Check sheet for the modelled part. Datum: model origin and axes. Units: mm. Face numbers are marked on the shaded views. A direction names the side the tool comes from. Round coordinates to 2 decimals unless told otherwise and drop trailing zeros. Loops run counter-clockwise (first coordinate to the right, second up) from the corner with the lowest first, then second, coordinate; pieces in that order, holes last. Notation, with made-up numbers: (-28.5, -39.75) -> (-9.5, -39.75) arc R5 ccw to (-9.5, -30.75) -> close; hole circle Ø6 at (11, 80.5). An arc over 180 degrees is marked (long way). One line per item, written item: value. Start each with the question number.
1. Material ranges on L1, parallel to X at y = -12.5, z = 43.5; L2, parallel to Y at x = 9, z = -55.5, recorded low to high.
2. Go/stop test with flat-tipped pins: pin 1 (1 mm diameter, centred on x = -9, y = 0, fed in from -Z); pin 2 (7.5 mm diameter, centred on y = 3.5, z = 45.5, fed in from -X); pin 3 (20.5 mm diameter, centred on x = -6.5, z = 53, fed in from -Y). Record where each tip stops, or that it passes through.
3. Cross-section at D-D on y = 7.5. Record the cut outline in (x, z), then the cut area to 3 significant figures.
4. Cross-section at B-B on y = -4. Record the cut outline in (x, z).
5. Cross-section at A-A on x = 0. Record the cut outline in (y, z), then the cut area to 3 significant figures.
6. Set-up check for the marked faces 1, 2, 3, 4 and 5: record each of +Z, -Z, +X, -X, +Y, -Y from which the full face is reachable in a straight line by a thin tool's end or side.
7. Cross-section at C-C on y = 17.5. Record the cut outline in (x, z).
8. Release check for a two-part mould opening along Z. For the marked faces 6, 7 and 8 record: +Z half, -Z half, draft (parallel to the pull), parting line (faces both ways), or undercut.
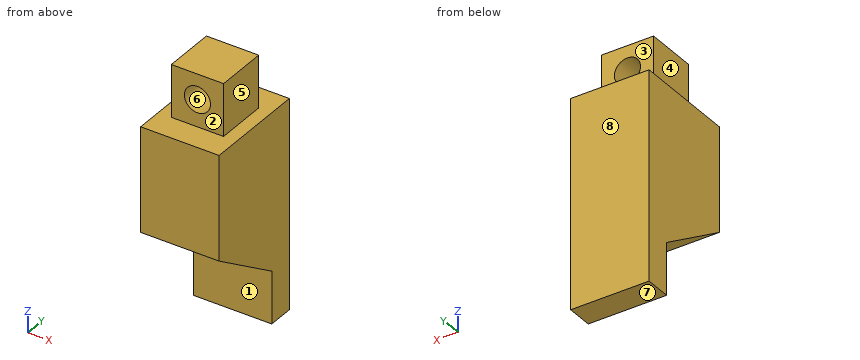
from build123d import *

# Parameters (mm, degrees)
F0_W     = 38.1
F0_H     = 76.2
F1_DEPTH = 25.4
F2_SIZE2 = 38.1
F2_SIZE  = 25.4
F3_W     = 25.4
F3_H     = 25.4
F4_DEPTH = 25.4
F5_R     = 6.35
F6_DEPTH = 25.4
F7_W     = 38.1
F7_H     = 12.7
F8_DEPTH = 25.4


with BuildPart() as f1:
    # F0 (on Front) → F1 (new body, symmetric)
    with BuildSketch(Plane.XZ):
        Rectangle(F0_W, F0_H)
    extrude(amount=F1_DEPTH, both=True)

    # F2
    f2_edges = [f1.edges().sort_by_distance(p)[0] for p in [
        (0, -25.4, -38.1),
    ]]
    chamfer(f2_edges, length=F2_SIZE, length2=F2_SIZE2)

    # F3 (on face) → F4 (join)
    with BuildSketch(Plane.XY.offset(38.1)):
        Rectangle(F3_W, F3_H)
    extrude(amount=F4_DEPTH)

    # F5 (on face) → F6 (cut)
    with BuildSketch(Plane.XZ.offset(12.7)):
        with Locations((0, 51.219936)):
            Circle(F5_R)
    extrude(amount=-F6_DEPTH, mode=Mode.SUBTRACT)

    # F7 (on face) → F8 (join)
    with BuildSketch(Plane(origin=(0, 0, -38.1), x_dir=(1, 0, 0), z_dir=(0, 0, -1))):
        with Locations((0, -19.05)):
            Rectangle(F7_W, F7_H)
    extrude(amount=F8_DEPTH)


solid = f1.part
Taken from the geometry:
1. L1: x = -12.7 to 12.7
1. L2: y = 12.7 to 25.4
2. pin 1: stops at z = -29.97
2. pin 2: stops at x = -12.7
2. pin 3: stops at y = -12.7
3. outline: (-19.05, -34.63) -> (19.05, -34.63) -> (19.05, 38.1) -> (12.7, 38.1) -> (12.7, 63.5) -> (-12.7, 63.5) -> (-12.7, 38.1) -> (-19.05, 38.1) -> close; hole circle Ø12.7 at (0, 51.22)
3. area: 3,290 mm2
4. outline: (-19.05, -26.97) -> (19.05, -26.97) -> (19.05, 38.1) -> (12.7, 38.1) -> (12.7, 63.5) -> (-12.7, 63.5) -> (-12.7, 38.1) -> (-19.05, 38.1) -> close; hole circle Ø12.7 at (0, 51.22)
5. outline: (-25.4, -12.7) -> (12.7, -38.1) -> (12.7, -63.5) -> (25.4, -63.5) -> (25.4, 38.1) -> (12.7, 38.1) -> (12.7, 44.87) -> (-12.7, 44.87) -> (-12.7, 38.1) -> (-25.4, 38.1) -> close; (-12.7, 57.57) -> (12.7, 57.57) -> (12.7, 63.5) -> (-12.7, 63.5) -> close
5. area: 4,030 mm2
6. face 1: -Z, +X, -X, -Y
6. face 2: +Z, +X, -X, -Y
6. face 3: +Z, +X, -X, +Y
6. face 4: +Z, -X, +Y, -Y
6. face 5: +Z, +X, +Y, -Y
7. outline: (-19.05, -63.5) -> (19.05, -63.5) -> (19.05, 38.1) -> (-19.05, 38.1) -> close
8. face 6: undercut
8. face 7: -Z half
8. face 8: draft
